from build123d import *

# Parameters (mm, degrees)
F1_DEPTH  = 60
F2_SIZE   = 40
F3_R      = 90
F4_DEPTH  = 10
F5_W      = 43
F5_H      = 43
F6_DEPTH  = 40
F7_R      = 4
F8_DEPTH  = 10
F9_W      = 126.410162
F9_H      = 60
F10_DEPTH = 50
F11_SIZE  = 40


with BuildPart() as f1:
    # F0 (on Top) → F1 (new body)
    with BuildSketch(Plane.XY):
        Polygon((-173.205081, -100), (173.205081, -100), (0, 200), align=None)
    extrude(amount=F1_DEPTH)

    # F2
    f2_edges = [f1.edges().sort_by_distance(p)[0] for p in [
        (-173.205081, -100, 30),
        (173.205081, -100, 30),
        (0, 200, 30),
    ]]
    chamfer(f2_edges, length=F2_SIZE)

    # F3 (on face) → F4 (join)
    with BuildSketch(Plane.XY.offset(60)):
        Circle(F3_R)
    extrude(amount=F4_DEPTH)

    # F5 (on face) → F6 (cut)
    with BuildSketch(Plane.XY.offset(60)):
        with Locations((0, 130.358984)):
            Rectangle(F5_W, F5_H)
        Polygon((-120.763738, -94.549038), (-83.524645, -73.049038), (-105.024645, -35.809946), (-142.263738, -57.309946), align=None)
        Polygon((142.263738, -57.309946), (105.024645, -35.809946), (83.524645, -73.049038), (120.763738, -94.549038), align=None)
    extrude(amount=-F6_DEPTH, mode=Mode.SUBTRACT)

    # F7 (on face) → F8 (cut)
    with BuildSketch(Plane.XY.offset(60)):
        with Locations((-29.5, 130.358984)):
            Circle(F7_R)
        with Locations((29.5, 130.358984)):
            Circle(F7_R)
        with Locations((-98.144192, -90.727241)):
            Circle(F7_R)
        with Locations((-127.644192, -39.631743)):
            Circle(F7_R)
        with Locations((127.644192, -39.631743)):
            Circle(F7_R)
        with Locations((98.144192, -90.727241)):
            Circle(F7_R)
    extrude(amount=-F8_DEPTH, mode=Mode.SUBTRACT)

    # F9 (on face) → F10 (join)
    with BuildSketch(Plane.XZ.offset(100)):
        with Locations((0, 30)):
            Rectangle(F9_W, F9_H)
    extrude(amount=F10_DEPTH)

    # F11
    f11_edges = [f1.edges().sort_by_distance(p)[0] for p in [
        (0, -150, 60),
    ]]
    chamfer(f11_edges, length=F11_SIZE)


solid = f1.part
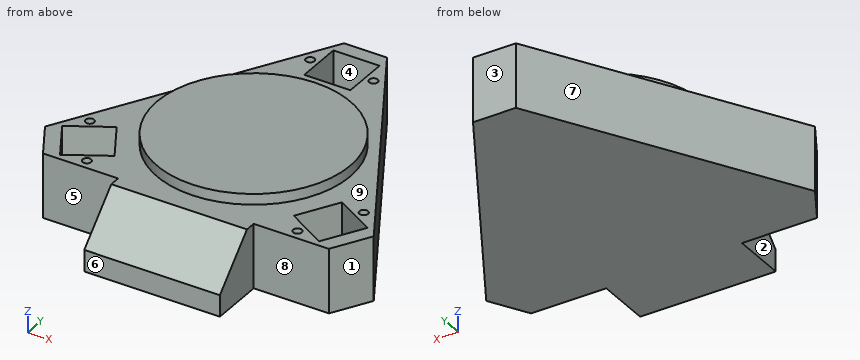
Work out the finished part from the listing and answer in its coordinate system (mm). Face numbers are marked on the shaded views. A direction names the side the tool comes from. Round coordinates to 2 decimals unless told otherwise and drop trailing zeros. Write each loop counter-clockwise with the first axis right and the second up, starting at its lowest first coordinate (ties: lowest second). Pieces come first, ordered by that corner, then holes. Notation, with made-up numbers: M 54.5,55 L 112.5,55 A17 cw 112.5,64 Z; hole C 75.25,-39 d11. An arc over 180 degrees is marked long. Use a Markdown table: item, result.
1) The part is cut by section C-C on z = 10. Give the vertices of the cut face in (x, y), plus the area to 3 significant figures.
Taken from the geometry:
| item | result |
|---|---|
| outline | M -153.21,-65.36 L -133.21,-100 L -63.21,-100 L -63.21,-150 L 63.21,-150 L 63.21,-100 L 133.21,-100 L 153.21,-65.36 L 20,165.36 L -20,165.36 Z |
| area | 56,200 mm2 |
2) The part is cut by section A-A on z = 42.5. Give the vertices of the cut face in (x, y), plus the area to 3 significant figures.
Taken from the geometry:
| item | result |
|---|---|
| outline | M -153.21,-65.36 L -133.21,-100 L -63.21,-100 L -63.21,-127.5 L 63.21,-127.5 L 63.21,-100 L 133.21,-100 L 153.21,-65.36 L 20,165.36 L -20,165.36 Z; hole M -142.26,-57.31 L -120.76,-94.55 L -83.52,-73.05 L -105.02,-35.81 Z; hole M -21.5,108.86 L 21.5,108.86 L 21.5,151.86 L -21.5,151.86 Z; hole M 83.52,-73.05 L 120.76,-94.55 L 142.26,-57.31 L 105.02,-35.81 Z |
| area | 47,800 mm2 |
3) The part is cut by section B-B on x = 0. Give the vertices of the cut face in (y, z), plus the area to 3 significant figures.
Taken from the geometry:
| item | result |
|---|---|
| outline | M -150,0 L 165.36,0 L 165.36,60 L 151.86,60 L 151.86,20 L 108.86,20 L 108.86,60 L 90,60 L 90,70 L -90,70 L -90,60 L -110,60 L -150,20 Z |
| area | 18,200 mm2 |
4) Which of the six approach directions +Z, -Z, +X, -X, +Y, -Y give full straight-line access (tool end or side, diameter ignored) to the marked faces 5, 6, 7, 8 and 9?
Taken from the geometry:
| item | result |
|---|---|
| face 5 | +Z, -Z, -X, -Y |
| face 6 | +Z, -Z, +X, -X, -Y |
| face 7 | +Z, -Z, -X, +Y |
| face 8 | +Z, -Z, +X, -Y |
| face 9 | +Z |
5) Flat-ended cylindrical pins translate along their axes: pin 1 (1.5 mm diameter, centred on x = 93, z = 49.5, fed in from -Y); pin 2 (2.5 mm diameter, centred on x = -128.5, y = -39, fed in from +Z); pin 3 (3 mm diameter, centred on y = 128, z = 26, fed in from +X); pin 4 (12 mm diameter, centred on x = 95, y = 59, fed in from -Z). Find the tip coordinate at first contact, or state that the pin passes through.
Taken from the geometry:
| item | result |
|---|---|
| pin 1 | stops at y = -100 |
| pin 2 | stops at z = 50 |
| pin 3 | stops at x = 42.44 |
| pin 4 | passes through |
6) The part is cut by section D-D on y = 0. Give the vertices of the cut face in (x, z).
Taken from the geometry:
| item | result |
|---|---|
| outline | M -115.47,0 L 115.47,0 L 115.47,60 L 90,60 L 90,70 L -90,70 L -90,60 L -115.47,60 Z |
7) Determine the mould class of the marked faces 1, 2, 3 and 4 for opening direction X: pulls with the +X half, pulls with the -X half, needs draft (parallel to the pull), parting line crosses it, or undercut.
Taken from the geometry:
| item | result |
|---|---|
| face 1 | pulls with the +X half |
| face 2 | pulls with the -X half |
| face 3 | needs draft |
| face 4 | undercut |
8) Consider line 1 (X direction, y = 124, z = 53); line 2 (X direction, y = -69, z = 48); line 3 (Z direction, x = 10.5, y = 119). Determine where each line is inside the solid, lowest interval first. Write a range as [from, to].
Taken from the geometry:
| item | result |
|---|---|
| line 1 | x = [-43.88, -21.5], [21.5, 43.88] |
| line 2 | x = [-151.1, -135.51], [-85.86, 85.86], [135.51, 151.1] |
| line 3 | z = [0, 20] |
